Could you check a few things on this drawing? It's one solid part, dimensions in mm from its lowest x, y, z. Coordinates: 2 decimals unless noted, no trailing zeros. Order: outer loops, then holes, each group sorted by start corner. A loop starts at its lowest first (then second) coordinate and runs counter-clockwise, first axis right, second up.
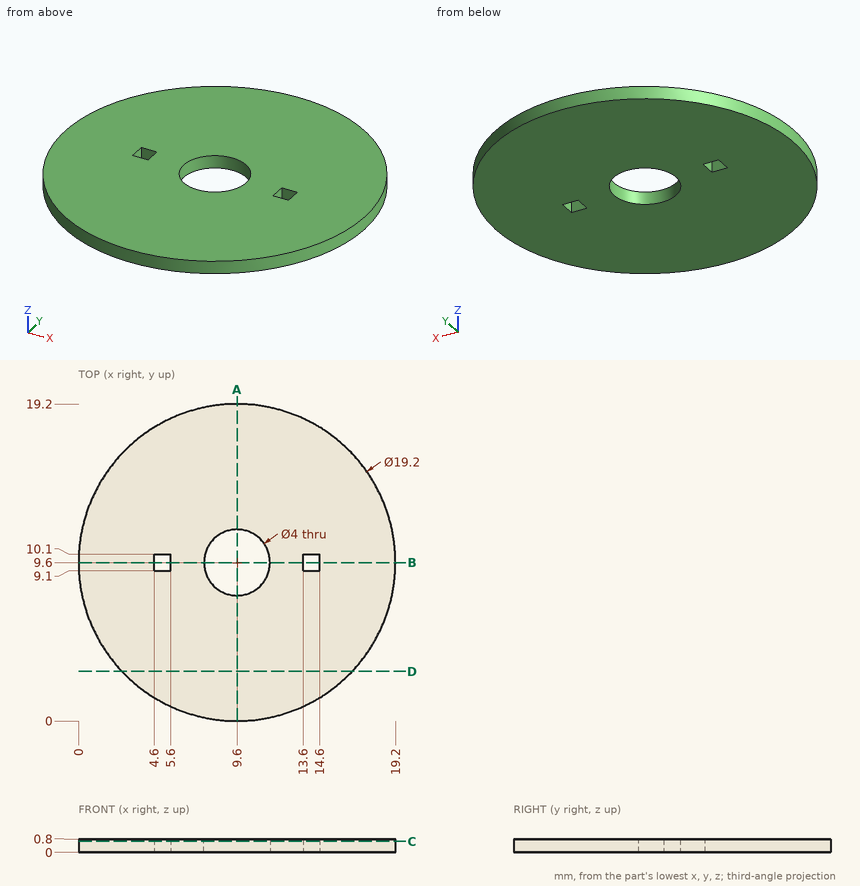
Q1. If we section it at D-D on y = 3: Write out the boundary of the cut face in (x, z).
Q2. If we section it at A-A on x = 9.6: Write out the boundary of the cut face in (y, z).
Q3. If we section it at C-C on z = 0.65: Write out the boundary of the cut face in (x, y).
Q4. If we section it at B-B on y = 9.6: Write out the boundary of the cut face in (x, z).
Q5. I need wall thicknesses on L1, parallel to Y at x = 9.6, z = 0.4; L2, parallel to X at y = 10, z = 0.4; L3, parallel to Y at x = 5, z = 0.55. Which ranges of each line are inside material? Lowest first, please.
Reply:
1. outline: (2.63, 0) - (16.57, 0) - (16.57, 0.8) - (2.63, 0.8) - close
2. outline: (0, 0) - (7.6, 0) - (7.6, 0.8) - (0, 0.8) - close; (11.6, 0) - (19.2, 0) - (19.2, 0.8) - (11.6, 0.8) - close
3. outline: circle Ø19.2 at (9.6, 9.6); hole (4.6, 9.1) - (5.6, 9.1) - (5.6, 10.1) - (4.6, 10.1) - close; hole circle Ø4 at (9.6, 9.6); hole (13.6, 9.1) - (14.6, 9.1) - (14.6, 10.1) - (13.6, 10.1) - close
4. outline: (0, 0) - (4.6, 0) - (4.6, 0.8) - (0, 0.8) - close; (5.6, 0) - (7.6, 0) - (7.6, 0.8) - (5.6, 0.8) - close; (11.6, 0) - (13.6, 0) - (13.6, 0.8) - (11.6, 0.8) - close; (14.6, 0) - (19.2, 0) - (19.2, 0.8) - (14.6, 0.8) - close
5. L1: y = 0 to 7.6, 11.6 to 19.2
5. L2: x = 0.01 to 4.6, 5.6 to 7.64, 11.56 to 13.6, 14.6 to 19.19
5. L3: y = 1.17 to 9.1, 10.1 to 18.03
